Check sheet for the modelled part. Datum: model origin and axes. Units: mm. A direction names the side the tool comes from. Round coordinates to 2 decimals unless told otherwise and drop trailing zeros. Loops run counter-clockwise (first coordinate to the right, second up) from the corner with the lowest first, then second, coordinate; pieces in that order, holes last. Notation, with made-up numbers: (-19.5, 31) - (35.5, 31) arc R17 cw to (35.5, 36) - close; hole circle Ø5 at (13.5, -6). An arc over 180 degrees is marked (long way). Return JSON: item names as keys, results as strings.
from build123d import *

# Parameters (mm, degrees)
F1_DEPTH = 3
F2_W     = 3
F2_H     = 3
F2_H_2   = 120
F3_DEPTH = 41
F5_DEPTH = 3
F7_DEPTH = 39.6


with BuildPart() as f1:
    # F0 (on Right) → F1 (new body)
    with BuildSketch(Plane.YZ):
        Polygon((-7, -20), (5, -20), (17, -20), (17, 100), (14, 109.5393920142), (-4, 109.5393920142), (-7, 100), align=None)
        with BuildLine():
            Line((10, 28), (10, 12))
            ThreePointArc((10, 12), (11.4142135624, 11.4142135624), (12, 10))
            ThreePointArc((12, 10), (11.4142135624, 8.5857864376), (10, 8))
            Line((10, 8), (10, 0))
            Line((10, 0), (5, 0))
            Line((5, 0), (2, 0))
            ThreePointArc((2, 0), (-1.4142135624, -1.4142135624), (0, 2))
            Line((0, 2), (0, 18))
            ThreePointArc((0, 18), (-2, 20), (0, 22))
            Line((0, 22), (0, 38))
            ThreePointArc((0, 38), (-2, 40), (0, 42))
            Line((0, 42), (0, 58))
            ThreePointArc((0, 58), (-2, 60), (0, 62))
            Line((0, 62), (0, 78))
            ThreePointArc((0, 78), (-2, 80), (0, 82))
            Line((0, 82), (0, 98))
            ThreePointArc((0, 98), (-1.4142135624, 101.4142135624), (2, 100))
            ThreePointArc((2, 100), (1.847759065, 99.2346331353), (1.4142135624, 98.5857864376))
            Line((1.4142135624, 98.5857864376), (8.5857864376, 91.4142135624))
            ThreePointArc((8.5857864376, 91.4142135624), (10.7653668647, 91.847759065), (12, 90))
            ThreePointArc((12, 90), (11.4142135624, 88.5857864376), (10, 88))
            Line((10, 88), (10, 72))
            ThreePointArc((10, 72), (11.4142135624, 71.4142135624), (12, 70))
            ThreePointArc((12, 70), (11.4142135624, 68.5857864376), (10, 68))
            Line((10, 68), (10, 52))
            ThreePointArc((10, 52), (11.4142135624, 51.4142135624), (12, 50))
            ThreePointArc((12, 50), (11.4142135624, 48.5857864376), (10, 48))
            Line((10, 48), (10, 32))
            ThreePointArc((10, 32), (11.4142135624, 31.4142135624), (12, 30))
            ThreePointArc((12, 30), (11.4142135624, 28.5857864376), (10, 28))
        make_face(mode=Mode.SUBTRACT)
        with BuildLine():
            ThreePointArc((8.5857864376, 8.5857864376), (8, 10), (8.5857864376, 11.4142135624))
            Line((8.5857864376, 11.4142135624), (1.4142135624, 18.5857864376))
            ThreePointArc((1.4142135624, 18.5857864376), (0.7653668647, 18.152240935), (0, 18))
            Line((0, 18), (0, 2))
            ThreePointArc((0, 2), (0.7653668647, 1.847759065), (1.4142135624, 1.4142135624))
            Line((1.4142135624, 1.4142135624), (8.5857864376, 8.5857864376))
        make_face()
        with BuildLine():
            ThreePointArc((10, 8), (9.2346331353, 8.152240935), (8.5857864376, 8.5857864376))
            Line((8.5857864376, 8.5857864376), (1.4142135624, 1.4142135624))
            ThreePointArc((1.4142135624, 1.4142135624), (1.847759065, 0.7653668647), (2, 0))
            Line((2, 0), (5, 0))
            Line((5, 0), (10, 0))
            Line((10, 0), (10, 8))
        make_face()
        with BuildLine():
            Line((1.4142135624, 18.5857864376), (8.5857864376, 11.4142135624))
            ThreePointArc((8.5857864376, 11.4142135624), (9.2346331353, 11.847759065), (10, 12))
            Line((10, 12), (10, 28))
            ThreePointArc((10, 28), (9.2346331353, 28.152240935), (8.5857864376, 28.5857864376))
            Line((8.5857864376, 28.5857864376), (1.4142135624, 21.4142135624))
            ThreePointArc((1.4142135624, 21.4142135624), (1.847759065, 20.7653668647), (2, 20))
            ThreePointArc((2, 20), (1.847759065, 19.2346331353), (1.4142135624, 18.5857864376))
        make_face()
        with BuildLine():
            Line((1.4142135624, 21.4142135624), (8.5857864376, 28.5857864376))
            ThreePointArc((8.5857864376, 28.5857864376), (8, 30), (8.5857864376, 31.4142135624))
            Line((8.5857864376, 31.4142135624), (1.4142135624, 38.5857864376))
            ThreePointArc((1.4142135624, 38.5857864376), (0.7653668647, 38.152240935), (0, 38))
            Line((0, 38), (0, 22))
            ThreePointArc((0, 22), (0.7653668647, 21.847759065), (1.4142135624, 21.4142135624))
        make_face()
        with BuildLine():
            Line((1.4142135624, 38.5857864376), (8.5857864376, 31.4142135624))
            ThreePointArc((8.5857864376, 31.4142135624), (9.2346331353, 31.847759065), (10, 32))
            Line((10, 32), (10, 48))
            ThreePointArc((10, 48), (9.2346331353, 48.152240935), (8.5857864376, 48.5857864376))
            Line((8.5857864376, 48.5857864376), (1.4142135624, 41.4142135624))
            ThreePointArc((1.4142135624, 41.4142135624), (1.847759065, 40.7653668647), (2, 40))
            ThreePointArc((2, 40), (1.847759065, 39.2346331353), (1.4142135624, 38.5857864376))
        make_face()
        with BuildLine():
            Line((0, 58), (0, 42))
            ThreePointArc((0, 42), (0.7653668647, 41.847759065), (1.4142135624, 41.4142135624))
            Line((1.4142135624, 41.4142135624), (8.5857864376, 48.5857864376))
            ThreePointArc((8.5857864376, 48.5857864376), (8, 50), (8.5857864376, 51.4142135624))
            Line((8.5857864376, 51.4142135624), (1.4142135624, 58.5857864376))
            ThreePointArc((1.4142135624, 58.5857864376), (0.7653668647, 58.152240935), (0, 58))
        make_face()
        with BuildLine():
            Line((1.4142135624, 58.5857864376), (8.5857864376, 51.4142135624))
            ThreePointArc((8.5857864376, 51.4142135624), (9.2346331353, 51.847759065), (10, 52))
            Line((10, 52), (10, 68))
            ThreePointArc((10, 68), (9.2346331353, 68.152240935), (8.5857864376, 68.5857864376))
            Line((8.5857864376, 68.5857864376), (1.4142135624, 61.4142135624))
            ThreePointArc((1.4142135624, 61.4142135624), (1.847759065, 60.7653668647), (2, 60))
            ThreePointArc((2, 60), (1.847759065, 59.2346331353), (1.4142135624, 58.5857864376))
        make_face()
        with BuildLine():
            Line((0, 78), (0, 62))
            ThreePointArc((0, 62), (0.7653668647, 61.847759065), (1.4142135624, 61.4142135624))
            Line((1.4142135624, 61.4142135624), (8.5857864376, 68.5857864376))
            ThreePointArc((8.5857864376, 68.5857864376), (8, 70), (8.5857864376, 71.4142135624))
            Line((8.5857864376, 71.4142135624), (1.4142135624, 78.5857864376))
            ThreePointArc((1.4142135624, 78.5857864376), (0.7653668647, 78.152240935), (0, 78))
        make_face()
        with BuildLine():
            ThreePointArc((2, 80), (1.847759065, 79.2346331353), (1.4142135624, 78.5857864376))
            Line((1.4142135624, 78.5857864376), (8.5857864376, 71.4142135624))
            ThreePointArc((8.5857864376, 71.4142135624), (9.2346331353, 71.847759065), (10, 72))
            Line((10, 72), (10, 88))
            ThreePointArc((10, 88), (9.2346331353, 88.152240935), (8.5857864376, 88.5857864376))
            Line((8.5857864376, 88.5857864376), (1.4142135624, 81.4142135624))
            ThreePointArc((1.4142135624, 81.4142135624), (1.847759065, 80.7653668647), (2, 80))
        make_face()
        with BuildLine():
            Line((0, 98), (0, 82))
            ThreePointArc((0, 82), (0.7653668647, 81.847759065), (1.4142135624, 81.4142135624))
            Line((1.4142135624, 81.4142135624), (8.5857864376, 88.5857864376))
            ThreePointArc((8.5857864376, 88.5857864376), (8, 90), (8.5857864376, 91.4142135624))
            Line((8.5857864376, 91.4142135624), (1.4142135624, 98.5857864376))
            ThreePointArc((1.4142135624, 98.5857864376), (0.7653668647, 98.152240935), (0, 98))
        make_face()
    extrude(amount=-F1_DEPTH)

    # F2 (on face) → F3 (join)
    with BuildSketch(Plane(origin=(-3, 0, 0), x_dir=(0, -1, 0), z_dir=(-1, 0, 0))):
        with Locations((-18.5, -21.5)):
            Rectangle(F2_W, F2_H)
        with Locations((-18.5, 40)):
            Rectangle(F2_W, F2_H_2)
        Polygon((7, 109.5393920142), (4, 109.5393920142), (7, 100), (7, -20), (7, -23), (10, -23), (10, 100), align=None)
        Polygon((-17, 100), (-14, 109.5393920142), (-17, 109.5393920142), (-20, 100), align=None)
    extrude(amount=-F3_DEPTH)

    # F4 (on face) → F5 (join)
    with BuildSketch(Plane.YZ.offset(38)):
        Polygon((17, 109.5393920142), (-7, 109.5393920142), (-10, 100), (-10, -23), (20, -23), (20, 100), align=None)
    extrude(amount=-F5_DEPTH)

    # F6 (on face) → F7 (cut)
    with BuildSketch(Plane(origin=(0, 20, 0), x_dir=(-1, 0, 0), z_dir=(0, 1, 0))):
        Polygon((3, 95.2), (3, 100), (3, 110), (-38, 110), (-38, 108.2), align=None)
    extrude(amount=-F7_DEPTH, mode=Mode.SUBTRACT)


solid = f1.part
Q1. Depth check by flat-ended pin: P1, Ø0.9, axis at x = -1.5, y = 5, coming from the -Z side. Enter the tip coordinate at first touch or a pass-through.
Answer key:
{"P1": "stops at z = -20"}
Q2. Draft check along Y on faces 5 (the face through (17, 20, 39)), 6 (the face through (28.49, -6.351, 102.064)), 7 (the face through (30.64, -9.3, 102.22)), 8 (the face through (-3, 5, 37)). Enter one of: released by +Y, released by -Y, zero draft, split by the parting line, or undercut.
Answer key:
{"face 5": "released by +Y", "face 6": "undercut", "face 7": "released by -Y", "face 8": "zero draft"}
Q3. Sectioned sample at C-C (z = 53.5). Enter the section's corners in (x, y), plus the area to 3 significant figures.
Answer key:
{"outline": "(-3, -10) - (38, -10) - (38, 20) - (-3, 20) - close; hole (0, -7) - (35, -7) - (35, 17) - (0, 17) - close", "area": "390 mm²"}
Q4. Scan lines: probe 1 along X at (y, z) = (5, -17); probe 2 along Y at (x, z) = (31, 11.5); probe 3 along Z at (x, y) = (-1.55, 0). Record each from-to range of solid material in increasing order. Write a range as [from, to].
Answer key:
{"probe 1": "x = [-3, 0], [35, 38]", "probe 2": "y = [-10, -7], [17, 20]", "probe 3": "z = [-20, -2], [2, 18], [22, 38], [42, 58], [62, 78], [82, 95.66]"}
Q5. Sectioned sample at A-A (y = 5). Enter the section's corners in (x, z).
Answer key:
{"outline": "(-3, -20) - (0, -20) - (0, 96.15) - (-3, 95.2) - close; (35, -23) - (38, -23) - (38, 108.2) - (35, 107.25) - close"}
Q6. Tool access check on faces 1 (the face through (0, 5, 39)), 2 (the face through (28.49, 16.383, 101.963)), 3 (the face through (20, -7, 39)), 4 (the face through (23.5, 17.3, -23)). Record the directions out of +Z, -Z, +X, -X, +Y, -Y that give a thin tool (end or side, any length) a straight path to the whole face; none if there is none.
Answer key:
{"face 1": "+Z, -Z", "face 2": "-Z, -X", "face 3": "-Z", "face 4": "-Z, +X, -X, +Y, -Y"}
Q7. Sectioned sample at D-D (x = 33). Enter the section's corners in (y, z), plus the area to 3 significant figures.
Answer key:
{"outline": "(-10, -23) - (-7, -23) - (-7, 100) - (-4.92, 106.61) - (-7.92, 106.61) - (-10, 100) - close; (14.92, 106.61) - (17, 100) - (17, -23) - (20, -23) - (20, 100) - (17.92, 106.61) - close", "area": "778 mm²"}
Q8. Sectioned sample at B-B (x = 8.5). Enter the section's corners in (y, z).
Answer key:
{"outline": "(-10, -23) - (-7, -23) - (-7, 98.85) - (-10, 98.85) - close; (17, -23) - (20, -23) - (20, 98.85) - (17, 98.85) - close"}
